Part model, mm, in its own coordinate system. Round coordinates to 2 decimals unless told otherwise and drop trailing zeros. Write each loop counter-clockwise with the first axis right and the second up, starting at its lowest first coordinate (ties: lowest second). Pieces come first, ordered by that corner, then holes. Notation, with made-up numbers: M 84,79.5 L 135,79.5 A20 ccw 135,112.5 Z; hole C 26,52 d9. An arc over 180 degrees is marked long. Use a Markdown table: item, result. Add a question column.
1) Slice it at B-B on z = 18. Write the cut outline in (x, y).
2) Slice it at A-A on x = 0. Write the cut outline in (y, z).
3) Wall check: probe 1 along X at (y, z) = (-0.1, 18); probe 2 along Z at (x, y) = (52.5, -2); probe 3 along X at (y, z) = (0.2, 17). Give the ranges that are in metal, low to high.
4) Slice it at D-D on y = -1.6. Give the number of separate pieces and of enclosed holes in the cut face, plus the area to 3 significant figures.
5) Slice it at C-C on x = 52. Write the cut outline in (y, z), plus the area to 3 significant figures.
6) Drop flat-ended pins along their axis: P1, Ø6, axis at x = -29.1, z = 10.72, coming from the +Y side; P2, Ø1, axis at x = 22, y = -1.5, coming from the +Z side (3 decimals); P3, Ø3, axis at x = -7.5, y = -1, coming from the +Z side. Give the stop position or say it passes through.
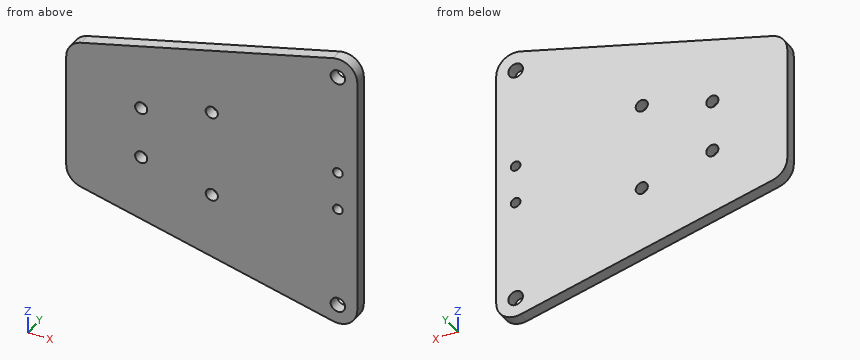
```python
from build123d import *

# Parameters (mm, degrees)
BOSS_EXTRUDE1_DEPTH = 2.5
SKETCH2_R           = 3
SKETCH2_R_2         = 2.5
SKETCH2_R_3         = 2
CUT_EXTRUDE1_DEPTH  = 5


with BuildPart() as part:
    # Sketch1 → Boss-Extrude1 (new, symmetric)
    with BuildSketch(Plane(origin=(0, 0, 0), x_dir=(1, 0, 0), z_dir=(0, 1, 0))):
        with BuildLine():
            Line((-60, -23.753788749), (-60, 23.753788749))
            ThreePointArc((-60, 23.753788749), (-58.305643504, 28.677086424), (-53.940285, 31.51492875))
            Line((-53.940285, 31.51492875), (50.059715, 57.51492875))
            ThreePointArc((50.059715, 57.51492875), (56.923297675, 56.059432253), (60, 49.753788749))
            Line((60, 49.753788749), (60, -49.753788749))
            ThreePointArc((60, -49.753788749), (56.923297675, -56.059432253), (50.059715, -57.51492875))
            Line((50.059715, -57.51492875), (-53.940285, -31.51492875))
            ThreePointArc((-53.940285, -31.51492875), (-58.305643504, -28.677086424), (-60, -23.753788749))
        make_face()
    extrude(amount=BOSS_EXTRUDE1_DEPTH, both=True)

    # Sketch2 → Cut-Extrude1 (cut)
    with BuildSketch(Plane(origin=(0, 2.5, 0), x_dir=(1, 0, 0), z_dir=(0, 1, 0))):
        with Locations(Location((52, 49.753788749, 0), (0, 0, 270))):
            Circle(SKETCH2_R)
        with Locations(Location((0, 18, 0), (0, 0, 270))):
            Circle(SKETCH2_R_2)
        with Locations(Location((52, -49.753788749, 0), (0, 0, 270))):
            Circle(SKETCH2_R)
        with Locations(Location((0, -18, 0), (0, 0, 270))):
            Circle(SKETCH2_R_2)
        with Locations(Location((-29.104275004, 10.723931249, 0), (0, 0, 270))):
            Circle(SKETCH2_R_2)
        with Locations(Location((-29.104275004, -10.723931249, 0), (0, 0, 270))):
            Circle(SKETCH2_R_2)
        with Locations(Location((52, 8, 0), (0, 0, 270))):
            Circle(SKETCH2_R_3)
        with Locations(Location((52, -8, 0), (0, 0, 270))):
            Circle(SKETCH2_R_3)
    extrude(amount=-CUT_EXTRUDE1_DEPTH, mode=Mode.SUBTRACT)


solid = part.part
```
Entries:
| question | item | result |
|---|---|---|
| 1 | outline | M -60,-2.5 L -2.5,-2.5 L -2.5,2.5 L -60,2.5 Z; M 2.5,-2.5 L 60,-2.5 L 60,2.5 L 2.5,2.5 Z |
| 2 | outline | M -2.5,-45 L 2.5,-45 L 2.5,-20.5 L -2.5,-20.5 Z; M -2.5,-15.5 L 2.5,-15.5 L 2.5,15.5 L -2.5,15.5 Z; M -2.5,20.5 L 2.5,20.5 L 2.5,45 L -2.5,45 Z |
| 3 | probe 1 | x = -60 to -2.5, 2.5 to 60 |
| 3 | probe 2 | z = -57.74 to -52.71, -46.8 to -9.94, -6.06 to 6.06, 9.94 to 46.8, 52.71 to 57.74 |
| 3 | probe 3 | x = -60 to -2.29, 2.29 to 60 |
| 4 | separate pieces | 1 |
| 4 | enclosed holes | 8 |
| 4 | area | 10,600 mm^2 |
| 5 | outline | M -2.5,-57.75 L 2.5,-57.75 L 2.5,-52.75 L -2.5,-52.75 Z; M -2.5,-46.75 L 2.5,-46.75 L 2.5,-10 L -2.5,-10 Z; M -2.5,-6 L 2.5,-6 L 2.5,6 L -2.5,6 Z; M -2.5,10 L 2.5,10 L 2.5,46.75 L -2.5,46.75 Z; M -2.5,52.75 L 2.5,52.75 L 2.5,57.75 L -2.5,57.75 Z |
| 5 | area | 478 mm^2 |
| 6 | P1 | stops at y = 2.5 |
| 6 | P2 | stops at z = 50.625 |
| 6 | P3 | stops at z = 43.5 |
